from build123d import *

# Parameters (mm, degrees)
F0_W      = 769
F0_H      = 696
F0_W_2    = 737
F0_H_2    = 664
F1_DEPTH  = 600
F2_W      = 737
F2_H      = 16
F3_DEPTH  = 86
F4_W      = 290
F4_H      = 400
F4_W_2    = 340
F5_DEPTH  = 110
F6_R      = 30
F7_W      = 737
F7_H      = 169
F8_DEPTH  = 16
F9_R      = 25
F10_DEPTH = 40
F11_R     = 25
F12_DEPTH = 40
F13_R     = 15
F14_ANGLE = 40


# Not quite as in the source:
# - a feature of the source that left no trace in its solid (it failed there, or was rolled back) is left out
# - a pattern or mirror of a feature is missing from the dataset's text; its kind, count and spacing are read off the source's solid


with BuildPart() as f1:
    # F0 (on Front) → F1 (new body)
    with BuildSketch(Plane.XZ):
        with Locations((368.5, 332)):
            Rectangle(F0_W, F0_H)
        with Locations((368.5, 332)):
            Rectangle(F0_W_2, F0_H_2, mode=Mode.SUBTRACT)
    extrude(amount=-F1_DEPTH)

    # F2 (on face) → F3 (join)
    with BuildSketch(Plane.XY):
        with Locations((368.5, 423)):
            Rectangle(F2_W, F2_H)
    extrude(amount=F3_DEPTH)

    # F4 (on face) → F5 (join)
    with BuildSketch(Plane(origin=(0, 0, 664), x_dir=(1, 0, 0), z_dir=(0, 0, -1))):
        with Locations((175, -232)):
            Rectangle(F4_W, F4_H)
        with Locations((540, -232)):
            Rectangle(F4_W_2, F4_H)
    extrude(amount=F5_DEPTH)

    # F6
    f6_edges = [f1.edges().sort_by_distance(p)[0] for p in [
        (175, 32, 554),
        (30, 232, 554),
        (175, 432, 554),
        (320, 232, 554),
        (540, 32, 554),
        (370, 232, 554),
        (540, 432, 554),
        (710, 232, 554),
    ]]
    fillet(f6_edges, radius=F6_R)

    # F7 (on face) → F8 (cut, through all)
    with BuildSketch(Plane.XY):
        with Locations((368.5, 515.5)):
            Rectangle(F7_W, F7_H)
    extrude(amount=-F8_DEPTH, mode=Mode.SUBTRACT)

    # F9 (on face) → F10 (join)
    with BuildSketch(Plane(origin=(0, 0, 554), x_dir=(1, 0, 0), z_dir=(0, 0, -1))):
        with Locations((175, -367)):
            Circle(F9_R)
    extrude(amount=F10_DEPTH)

    # F11 (on face) → F12 (join)
    with BuildSketch(Plane(origin=(0, 0, 554), x_dir=(1, 0, 0), z_dir=(0, 0, -1))):
        with Locations((450, -367)):
            Circle(F11_R)
    extrude(amount=F12_DEPTH)

    # F13 (on face) → F14 (revolve)
    with BuildSketch(Plane(origin=(0, 0, 514), x_dir=(1, 0, 0), z_dir=(0, 0, -1))):
        with Locations((450, -367)):
            Circle(F13_R)
    f14 = revolve(axis=Axis((540, 402, 554), (1, 0, 0)), revolution_arc=F14_ANGLE)

    # F14_copies: F14 across plane
    add(f14.mirror(Plane(origin=(312.5, 0, 0), x_dir=(0, 0, -1), z_dir=(-1, 0, 0))))


solid = f1.part
Read the model definition and answer for the solid it produces. Units are mm, in the model's axes. A direction names the side the tool comes from. Give positions to 0.01 mm unless a question says otherwise; leave off trailing zeros. Loops run counter-clockwise (first coordinate to the right, second up) from the corner with the lowest first, then second, coordinate; pieces in that order, holes last. Notation, with made-up numbers: M 50,-38 L 80,-38 A30 ccw 80,-9 Z; hole C 54,-25 d5. An arc over 180 degrees is marked long. Write each question's results on one line, items separated by ' | '.
1. Section D-D on y = 551.5 is taken. Give the vertices of the cut face in (x, z).
Values:
outline: M -16,-16 L 0,-16 L 0,664 L 737,664 L 737,-16 L 753,-16 L 753,680 L -16,680 Z
2. The mould has two halves that part along Z. Classify faces 1 (the face through (173, 432, 625)), 2 (the face through (363, 229, -16)), 3 (the face through (173, 230, 554)): pulls with the +Z half, pulls with the -Z half, needs draft (parallel to the pull), parting line crosses it, or undercut.
Values:
face 1: needs draft | face 2: pulls with the -Z half | face 3: undercut
3. Straight lines are drawn through the part: line 1 (X direction, y = 139.5, z = 388.5); line 2 (Z direction, x = 346, y = 69); line 3 (Z direction, x = 58, y = 207). For each, find the intervals that lie inside material, in ascending order. Write a range as [from, to].
Values:
line 1: x = [-16, 0], [737, 753] | line 2: z = [-16, 0], [664, 680] | line 3: z = [-16, 0], [554.07, 680]
4. Section C-C on y = 181 is taken. Give the vertices of the cut face in (x, z).
Values:
outline: M -16,-16 L 753,-16 L 753,680 L -16,680 Z; hole M 0,0 L 737,0 L 737,664 L 710,664 L 710,584 A30 cw 680,554 L 400,554 A30 cw 370,584 L 370,664 L 320,664 L 320,584 A30 cw 290,554 L 60,554 A30 cw 30,584 L 30,664 L 0,664 Z
5. Section B-B on x = 611 is taken. Give the vertices of the cut face in (y, z), plus the area to 3 significant figures.
Values:
outline: M 0,-16 L 431,-16 L 431,86 L 415,86 L 415,0 L 0,0 Z; M 0,664 L 32,664 L 32,584 A30 ccw 62,554 L 402,554 A30 ccw 432,584 L 432,664 L 600,664 L 600,680 L 0,680 Z | area: 61,500 mm^2
6. A tool of negligible diameter and unlimited length cuts with its end or side. For faces 4 (the face through (177.03, 423.445, 563.021)), 5 (the face through (538, 32, 625)), 6 (the face through (538, 432, 625)), 7 (the face through (378.555, 229.2, 563.021)), 8 (the face through (463.44, 345.92, 534.28)), from which of +Z, -Z, +X, -X, +Y, -Y can it reach the whole face along a straight path? Write none if from no direction.
Values:
face 4: +Y | face 5: -Y | face 6: -Z, +Y | face 7: +Y, -Y | face 8: none
7. Given pin 1 (24 mm diameter, centred on x = 214, z = 624.5, fed in from +Y), flat-ended and moving along its own axis, determine where the tip first touches the part or whether it passes through.
Values:
pin 1: stops at y = 432
8. Section A-A on z = 293 is taken. Give the vertices of the cut face in (x, y), plus the area to 3 significant figures.
Values:
outline: M -16,0 L 0,0 L 0,600 L -16,600 Z; M 737,0 L 753,0 L 753,600 L 737,600 Z | area: 19,200 mm^2
